Work out the finished part from the listing and answer in its coordinate system (mm). A direction names the side the tool comes from. Round coordinates to 2 decimals unless told otherwise and drop trailing zeros. Order: outer loops, then holes, each group sorted by start corner. A loop starts at its lowest first (then second) coordinate and runs counter-clockwise, first axis right, second up. Notation, with made-up numbers: M 89,74 L 148,74 A23 ccw 148,90 Z; hole C 68,-16 d6. An arc over 180 degrees is marked long. Return JSON: item names as keys, results as strings.
from build123d import *

# Parameters (mm, degrees)
F0_W     = 1.5
F0_H     = 98
F2_SIZE  = 0.5
F3_R     = 2.5
F3_R_2   = 1.5
F4_DEPTH = 2
F5_SIZE  = 0.5


with BuildPart() as f1:
    # F0 (on Right) → F1 (revolve)
    with BuildSketch(Plane.YZ):
        with Locations((-0.75, 0)):
            Rectangle(F0_W, F0_H)
    revolve(axis=Axis((0, 0, 0), (0, 0, -1)))

    # F2
    f2_edges = [f1.edges().sort_by_distance(p)[0] for p in [
        (0, 1.5, -49),
    ]]
    chamfer(f2_edges, length=F2_SIZE)

    # F3 (on face) → F4 (join)
    with BuildSketch(Plane.XY.offset(49)):
        Circle(F3_R)
        Circle(F3_R_2, mode=Mode.SUBTRACT)
        Circle(F3_R_2)
    extrude(amount=F4_DEPTH)

    # F5
    f5_edges = [f1.edges().sort_by_distance(p)[0] for p in [
        (-2.5, 0, 51),
    ]]
    chamfer(f5_edges, length=F5_SIZE)


solid = f1.part
Item 1: Which of the six approach directions +Z, -Z, +X, -X, +Y, -Y give full straight-line access (tool end or side, diameter ignored) to faces 1 (the cylindrical face through (-0.54, -2.44, 49.74)), 2 (the flat face through (0, -2, 49))?
Output:
{"face 1": "+Z, -Z", "face 2": "-Z"}
Item 2: Find section A-A (x = 0). Determine the outline of the cut face in (y, z), plus the area to 4 significant figures.
Output:
{"outline": "M -2.5,49 L -1.5,49 L -1.5,-48.5 L -1,-49 L 1,-49 L 1.5,-48.5 L 1.5,49 L 2.5,49 L 2.5,50.5 L 2,51 L -2,51 L -2.5,50.5 Z", "area": "303.5 mm^2"}
Item 3: Each of these flat-tipped pins is pushed along its axis until it touches: pin 1 (1.5 mm diameter, centred on y = 0.5, z = -12, fed in from +X); pin 2 (2 mm diameter, centred on y = -1, z = 3, fed in from -X); pin 3 (2 mm diameter, centred on x = 0.5, z = -13.5, fed in from -Y). Where does it stop, or does it pass through?
Output:
{"pin 1": "stops at x = 1.5", "pin 2": "stops at x = -1.5", "pin 3": "stops at y = -1.5"}
Item 4: Consider line 1 along Z through (x, y) = (0.8, 1.7); line 2 along Y through (x, z) = (0.65, -9); line 3 along X through (y, z) = (-0.05, -27). Determine where each line is inside the solid, lowest interval first. Write a range as [from, to].
Output:
{"line 1": "z = [49, 51]", "line 2": "y = [-1.35, 1.35]", "line 3": "x = [-1.5, 1.5]"}
Item 5: Find section C-C (z = 39.5). Determine the outline of the cut face in (x, y).
Output:
{"outline": "C 0,0 d3"}
